```python
from build123d import *

# Parameters (mm, degrees)
BOSS_EXTRUDE1_DEPTH = 3.175
FILLET1_R           = 3.175
SKETCH2_R           = 0.712880647
BOSS_EXTRUDE2_DEPTH = 2.54


with BuildPart() as part:
    # Sketch1 → Boss-Extrude1 (new body)
    with BuildSketch(Plane(origin=(0, 0, 0), x_dir=(1, 0, 0), z_dir=(0, 1, 0))):
        Polygon((0, 0), (-68.386624181, 46.529866421), (81.613375819, 46.529866421), align=None)
    extrude(amount=BOSS_EXTRUDE1_DEPTH)

    # Fillet1
    fillet1_edges = [part.edges().sort_by_distance(p)[0] for p in [
        (0, 1.5875, 0),
        (-68.386624181, 1.5875, -46.529866421),
        (81.613375819, 1.5875, -46.529866421),
    ]]
    fillet(fillet1_edges, radius=FILLET1_R)

    # Sketch2 → Boss-Extrude2 (add)
    with BuildSketch(Plane(origin=(0, 3.175, 0), x_dir=(1, 0, 0), z_dir=(0, 1, 0))):
        with Locations((-58.076097719, 43.354866421)):
            Circle(SKETCH2_R)
    extrude(amount=-BOSS_EXTRUDE2_DEPTH)


solid = part.part
```
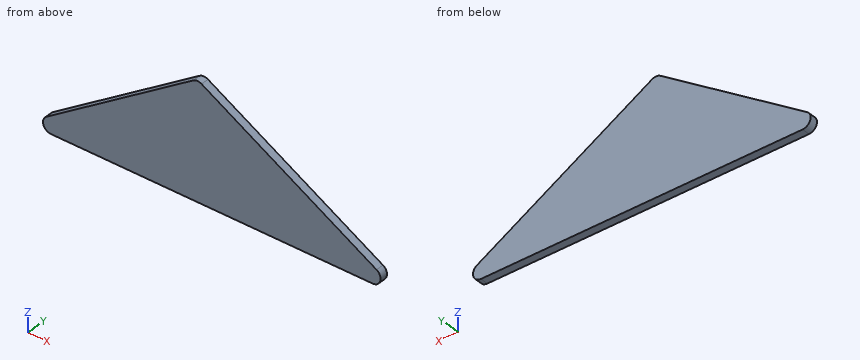
Input: part model. Units: mm. Frame: model coordinates. Round coordinates to 2 decimals unless told otherwise and drop trailing zeros. Order: outer loops, then holes, each group sorted by start corner. A loop starts at its lowest first (then second) coordinate and runs counter-clockwise, first axis right, second up. Notation, with made-up numbers: (-1, 73.25) - (54, 73.25) arc R21 cw to (54, 102.25) - close; hole circle Ø8 at (42.5, 45). An arc over 180 degrees is marked (long way). Answer in a Markdown table with one row per item.
Item 1: Section query A-A (y = 1.45). Return the cut outline in (x, z) (3 decimals).
Model answer:
| item | result |
|---|---|
| outline | (-59.862, -40.73) arc R3.175 ccw to (-58.076, -46.53) - (69.634, -46.53) arc R3.175 ccw to (71.207, -40.597) - (1.721, -0.981) arc R3.175 ccw to (-1.638, -1.114) - close |
Item 2: Section query C-C (x = -15). Return the cut outline in (y, z) (3 decimals).
Model answer:
| item | result |
|---|---|
| outline | (0, -46.53) - (3.175, -46.53) - (3.175, -10.206) - (0, -10.206) - close |
Item 3: Section query B-B (z = -23). Return the cut outline in (x, y) (3 decimals).
Model answer:
| item | result |
|---|---|
| outline | (-33.804, 0) - (40.342, 0) - (40.342, 3.175) - (-33.804, 3.175) - close |
Item 4: Pin query (flat end, axial travel): pin 1 (1.5 mm diameter, centred on y = 2, z = -23, fed in from +X). Return the tip coordinate at first contact, or that it passes through.
Model answer:
| item | result |
|---|---|
| pin 1 | stops at x = 41.66 |
Item 5: Line query: line 1 (X direction, y = 1.2, z = -38.5); line 2 (X direction, y = 1.75, z = -16); line 3 (Z direction, x = 24.5, y = 3). Output: solid intervals per line, ascending.
Model answer:
| item | result |
|---|---|
| line 1 | x = -56.58 to 67.53 |
| line 2 | x = -23.52 to 28.06 |
| line 3 | z = -46.53 to -13.97 |
